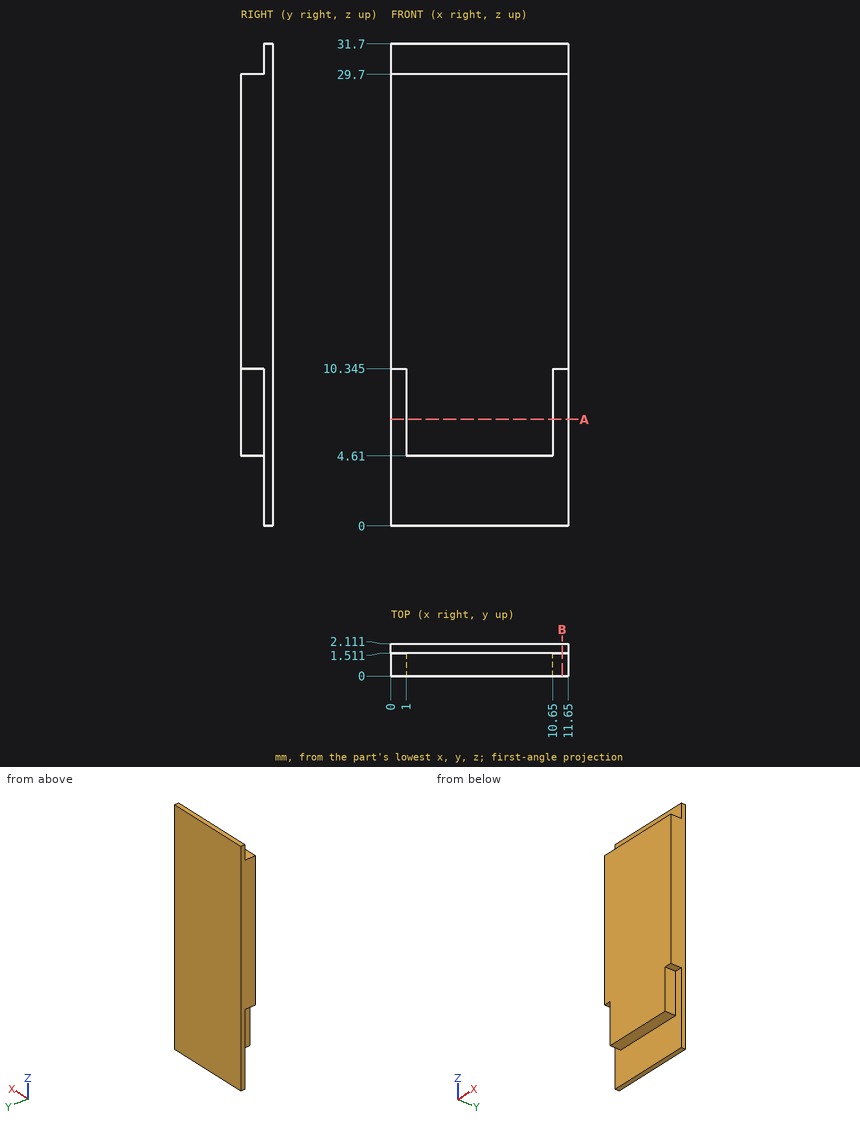
The drawing under review shows one solid part. Ordinate dimensions are in mm from its lowest x, y, z. Round coordinates to 2 decimals unless told otherwise and drop trailing zeros. Loops run counter-clockwise (first coordinate to the right, second up) from the corner with the lowest first, then second, coordinate; pieces in that order, holes last. Notation, with made-up numbers: (61.5, 39) - (74.5, 39) arc R33 cw to (74.5, 69) - close; hole circle Ø10 at (51, 11). An arc over 180 degrees is marked (long way). Use a Markdown table: item, result. Add a question column.
Q1. Add section A-A (z = 7). State the section outline as (x, y) points, plus the area to 3 significant figures.
Q2. Insertion check: pin 1 Ø0.8 at (x, y) = (0.5, 0.5) entering from -Z (3 decimals); pin 2 Ø1 at (x, z) = (7, 31) entering from -Y; pin 3 Ø0.5 at (y, z) = (0.5, 7.5) entering from -X. Each pin has a flat end and moves straight along its axis. Give the tip position at first contact, or say it passes through.
Q3. For probe 1 along Z at (x, y) = (3.75, 1.15); probe 2 along Y at (x, z) = (9.75, 2.5); probe 3 along Z at (x, y) = (0.5, 1.2) (1 decimal), list the stretches that pass through material, from the lowest coordinate up.
Q4. Add section B-B (x = 11.25). State the section outline as (y, z) points (1 decimal).
Worked answers:
| question | item | result |
|---|---|---|
| 1 | outline | (0, 1.51) - (1, 1.51) - (1, 0) - (10.65, 0) - (10.65, 1.51) - (11.65, 1.51) - (11.65, 2.11) - (0, 2.11) - close |
| 1 | area | 21.6 mm² |
| 2 | pin 1 | z = 10.345 |
| 2 | pin 2 | y = 1.51 |
| 2 | pin 3 | x = 1 |
| 3 | probe 1 | 4.61 to 29.7 |
| 3 | probe 2 | 1.51 to 2.11 |
| 3 | probe 3 | 10.3 to 29.7 |
| 4 | outline | (0, 10.3) - (1.5, 10.3) - (1.5, 0) - (2.1, 0) - (2.1, 31.7) - (1.5, 31.7) - (1.5, 29.7) - (0, 29.7) - close |
